Part model, mm, in its own coordinate system. A direction names the side the tool comes from. Give positions to 0.01 mm unless a question says otherwise; leave off trailing zeros. Order: outer loops, then holes, each group sorted by start corner. A loop starts at its lowest first (then second) coordinate and runs counter-clockwise, first axis right, second up. Notation, with made-up numbers: (5.5, 68) -> (30.5, 68) arc R16 cw to (30.5, 77) -> close; hole circle Ø9 at (38, 72.25). An arc over 180 degrees is marked (long way). Write item = value, one per line. Start each with the question number.
(1) Saw through at D-D, the plane z = 2.5. List the corners of the cut face in (x, y).
(2) Two-plate mould, pull along Z, no slides. Class faces 6 (the flat face through (-5, -4, -0.5)), 7 (the flat face through (-2.2, 3.5, -1.5)), 8 (the cylindrical face through (-0.689, -6.887, 0.837)), 9 (the flat face through (0, -6, 2)): pulls with the +Z half, pulls with the -Z half, needs draft (parallel to the pull), parting line crosses it, or undercut.
(3) Saw through at C-C, the plane y = 3.5. List the corners of the cut face in (x, z).
(4) Saw through at B-B, the plane x = -5. List the corners of the cut face in (y, z), then the cut area to 3 significant figures.
(5) Saw through at A-A, the plane z = -2. List the corners of the cut face in (x, y).
(6) Probe line 1 along X through (y, z) = (-6.5, 2.5); line 2 along Z through (x, y) = (0, -7.3); line 3 along Y through (x, z) = (0.5, -0.25). List the from-to ranges inside material, lowest first. Write a range as from..to.
(7) Flat gauge pins, fed straight in: pin 1 (0.8 mm diameter, centred on y = 3.5, z = -1, fed in from +X); pin 2 (0.8 mm diameter, centred on y = 3.5, z = -2, fed in from -X); pin 3 (1.3 mm diameter, centred on x = 0, y = 3.5, fed in from -Z). Where does each tip first touch, or does it go through?
(8) Which spindle directions (+Z, -Z, +X, -X, +Y, -Y) get a long thin tool onto all of the face, cutting with end or side? Do faces 1 (the flat face through (-5.3, 3.5, -1.5)), 2 (the flat face through (2.8, 3.5, -1.5)), 3 (the flat face through (5, -4, -0.5)), 4 (the flat face through (0, -1.2, -1)), 5 (the flat face through (5, -1.5, -0.5)). Say none if no direction does.
from build123d import *

# Parameters (mm, degrees)
SKETCH1_W                = 12
SKETCH1_H                = 12
BOSS_EXTRUDE1_DEPTH      = 5
BOSS_EXTRUDE2_DEPTH      = 2
BOSS_EXTRUDE2_DEPTH_BACK = 1
SKETCH2_R                = 3
SKETCH2_R_2              = 1.8
FILLET1_R                = 0.2
SKETCH3_R                = 0.6
BOSS_EXTRUDE3_DEPTH      = 0.5
BOSS_EXTRUDE4_DEPTH      = 3


with BuildPart() as part:
    # Sketch1 → Boss-Extrude1 (new body)
    with BuildSketch(Plane.XY):
        Rectangle(SKETCH1_W, SKETCH1_H)
    extrude(amount=BOSS_EXTRUDE1_DEPTH)

    # Sketch2 → Boss-Extrude2 (add, two sides: drawn at the far end of the back side and taken through both)
    with BuildSketch(Plane.XZ.offset(6).offset(-BOSS_EXTRUDE2_DEPTH_BACK)):
        with Locations(Location((0, 2.5, 0), (0, 0, 270))):
            Circle(SKETCH2_R)
        with Locations(Location((0, 2.5, 0), (0, 0, 270))):
            Circle(SKETCH2_R_2, mode=Mode.SUBTRACT)
    extrude(amount=BOSS_EXTRUDE2_DEPTH + BOSS_EXTRUDE2_DEPTH_BACK)

    # Fillet1
    fillet1_edges = [part.edges().sort_by_distance(p)[0] for p in [
        (0, -8, 4.3),
        (0, -8, 5.5),
    ]]
    fillet(fillet1_edges, radius=FILLET1_R)

    # Sketch3 → Boss-Extrude3 (add)
    with BuildSketch(Plane(origin=(0, 0, 0), x_dir=(-1, 0, 0), z_dir=(0, 0, -1))):
        with Locations((-5, -4)):
            Circle(SKETCH3_R)
        with Locations((5, -1.5)):
            Circle(SKETCH3_R)
        with Locations((5, -4)):
            Circle(SKETCH3_R)
        with Locations((0, 3.5)):
            Circle(SKETCH3_R)
        with Locations((-5, -1.5)):
            Circle(SKETCH3_R)
    extrude(amount=BOSS_EXTRUDE3_DEPTH)

    # Sketch3_3 → Boss-Extrude4 (add)
    with BuildSketch(Plane(origin=(0, 0, 0), x_dir=(-1, 0, 0), z_dir=(0, 0, -1))):
        with BuildLine():
            Line((-0.5, -1.2), (0.5, -1.2))
            ThreePointArc((0.5, -1.2), (0.8, -1.5), (0.5, -1.8))
            Line((0.5, -1.8), (-0.5, -1.8))
            ThreePointArc((-0.5, -1.8), (-0.8, -1.5), (-0.5, -1.2))
        make_face()
        with BuildLine():
            Line((-4.7, 4), (-4.7, 3))
            ThreePointArc((-4.7, 3), (-5, 2.7), (-5.3, 3))
            Line((-5.3, 3), (-5.3, 4))
            ThreePointArc((-5.3, 4), (-5, 4.3), (-4.7, 4))
        make_face()
        with BuildLine():
            Line((-2.2, 4), (-2.2, 3))
            ThreePointArc((-2.2, 3), (-2.5, 2.7), (-2.8, 3))
            Line((-2.8, 3), (-2.8, 4))
            ThreePointArc((-2.8, 4), (-2.5, 4.3), (-2.2, 4))
        make_face()
        with BuildLine():
            Line((4.7, 4), (4.7, 3))
            ThreePointArc((4.7, 3), (5, 2.7), (5.3, 3))
            Line((5.3, 3), (5.3, 4))
            ThreePointArc((5.3, 4), (5, 4.3), (4.7, 4))
        make_face()
        with BuildLine():
            Line((2.2, 4), (2.2, 3))
            ThreePointArc((2.2, 3), (2.5, 2.7), (2.8, 3))
            Line((2.8, 3), (2.8, 4))
            ThreePointArc((2.8, 4), (2.5, 4.3), (2.2, 4))
        make_face()
    extrude(amount=BOSS_EXTRUDE4_DEPTH)


solid = part.part
Results list:
q1.outline = (-6, -6) -> (-3, -6) -> (-3, -7.8) arc R0.2 ccw to (-2.8, -8) -> (-2, -8) arc R0.2 ccw to (-1.8, -7.8) -> (-1.8, -6) -> (1.8, -6) -> (1.8, -7.8) arc R0.2 ccw to (2, -8) -> (2.8, -8) arc R0.2 ccw to (3, -7.8) -> (3, -6) -> (6, -6) -> (6, 6) -> (-6, 6) -> close
q2.face_6 = pulls with the -Z half
q2.face_7 = needs draft
q2.face_8 = undercut
q2.face_9 = undercut
q3.outline = (-6, 0) -> (-5.3, 0) -> (-5.3, -3) -> (-4.7, -3) -> (-4.7, 0) -> (-2.8, 0) -> (-2.8, -3) -> (-2.2, -3) -> (-2.2, 0) -> (-0.6, 0) -> (-0.6, -0.5) -> (0.6, -0.5) -> (0.6, 0) -> (2.2, 0) -> (2.2, -3) -> (2.8, -3) -> (2.8, 0) -> (4.7, 0) -> (4.7, -3) -> (5.3, -3) -> (5.3, 0) -> (6, 0) -> (6, 5) -> (-6, 5) -> close
q4.outline = (-6, 0) -> (-4.6, 0) -> (-4.6, -0.5) -> (-3.4, -0.5) -> (-3.4, 0) -> (-2.1, 0) -> (-2.1, -0.5) -> (-0.9, -0.5) -> (-0.9, 0) -> (2.7, 0) -> (2.7, -3) -> (4.3, -3) -> (4.3, 0) -> (6, 0) -> (6, 5) -> (-6, 5) -> close
q4.area = 66.0 mm^2
q5.outline = (-5.3, 3) arc R0.3 ccw to (-4.7, 3) -> (-4.7, 4) arc R0.3 ccw to (-5.3, 4) -> close; (-2.8, 3) arc R0.3 ccw to (-2.2, 3) -> (-2.2, 4) arc R0.3 ccw to (-2.8, 4) -> close; (-0.5, -1.8) -> (0.5, -1.8) arc R0.3 ccw to (0.5, -1.2) -> (-0.5, -1.2) arc R0.3 ccw to start; (2.2, 3) arc R0.3 ccw to (2.8, 3) -> (2.8, 4) arc R0.3 ccw to (2.2, 4) -> close; (4.7, 3) arc R0.3 ccw to (5.3, 3) -> (5.3, 4) arc R0.3 ccw to (4.7, 4) -> close
q6.line_1 = -3..-1.8, 1.8..3
q6.line_2 = -0.5..0.7, 4.3..5.5
q6.line_3 = -8..-5, -1.8..-1.2, 3.17..3.83
q7.pin_1 = 5.3
q7.pin_2 = -5.3
q7.pin_3 = -0.5
q8.face_1 = -Z, -X, +Y
q8.face_2 = -Z, +Y, -Y
q8.face_3 = -Z, +X, -X, -Y
q8.face_4 = -Z
q8.face_5 = -Z, +X, -Y
